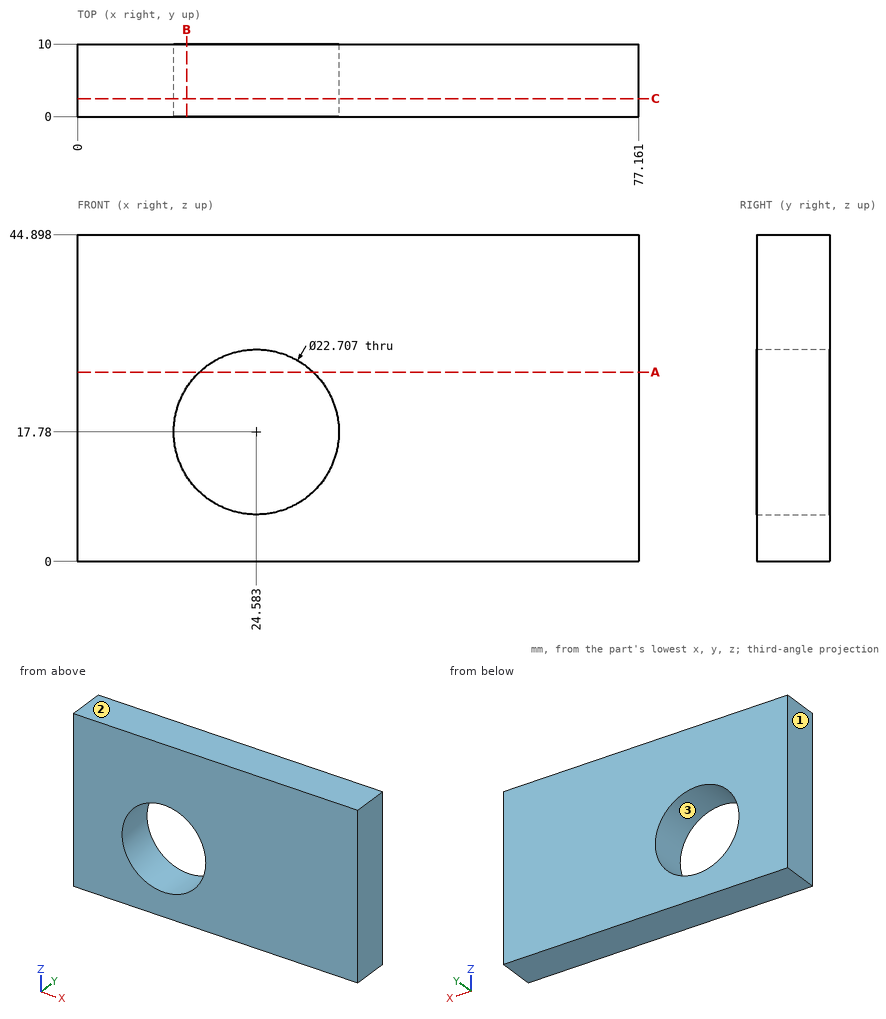
Print and shaded views of the part. All mm, measured from the part's lowest x, y and z. Round coordinates to 2 decimals unless told otherwise and drop trailing zeros. Order: outer loops, then holes, each group sorted by start corner. A loop starts at its lowest first (then second) coordinate and runs counter-clockwise, first axis right, second up. Notation, with made-up numbers: (42, -20.75) - (96, -20.75) arc R16 ccw to (96, -7.75) - close; hole circle Ø5 at (36, 10.5). An arc over 180 degrees is marked (long way). Use a Markdown table: item, result.
1) Saw through at B-B on x = 15. Write the cut outline in (y, z).
Recorded:
| item | result |
|---|---|
| outline | (0, 0) - (10, 0) - (10, 11.69) - (0, 11.69) - close; (0, 23.87) - (10, 23.87) - (10, 44.9) - (0, 44.9) - close |
2) Wall check: L1, parallel to X at y = 2.75, z = 17.5; L2, parallel to Z at x = 24.5, y = 7.5; L3, parallel to X at y = 2, z = 15 (1 decimal). Give the ranges that are in metal, low to high.
Recorded:
| item | result |
|---|---|
| L1 | x = 0 to 13.23, 35.93 to 77.16 |
| L2 | z = 0 to 6.43, 29.13 to 44.9 |
| L3 | x = 0 to 13.6, 35.6 to 77.2 |
3) Saw through at C-C on y = 2.5. Write the cut outline in (x, z), and give its area (3 significant figures).
Recorded:
| item | result |
|---|---|
| outline | (0, 0) - (77.16, 0) - (77.16, 44.9) - (0, 44.9) - close; hole circle Ø22.71 at (24.58, 17.78) |
| area | 3,060 mm² |
4) Pull direction Z, two halves, no side cores. Call the marked faces 1, 2 and 3: pulls with the +Z half, pulls with the -Z half, needs draft (parallel to the pull), parting line crosses it, or undercut.
Recorded:
| item | result |
|---|---|
| face 1 | needs draft |
| face 2 | pulls with the +Z half |
| face 3 | undercut |
5) Saw through at A-A on z = 26. Write the cut outline in (x, y) (1 decimal), and give its area (3 significant figures).
Recorded:
| item | result |
|---|---|
| outline | (0, 0) - (16.8, 0) - (16.8, 10) - (0, 10) - close; (32.4, 0) - (77.2, 0) - (77.2, 10) - (32.4, 10) - close |
| area | 615 mm² |
